Could you check a few things on this model? Use its own coordinates, in mm. A direction names the side the tool comes from. Round coordinates to 2 decimals unless told otherwise and drop trailing zeros. Loops run counter-clockwise (first coordinate to the right, second up) from the corner with the lowest first, then second, coordinate; pieces in that order, holes last.
from build123d import *

# Parameters (mm, degrees)
SKETCH1_W           = 100
SKETCH1_H           = 100
BOSS_EXTRUDE1_DEPTH = 10
SKETCH2_R           = 2.5
CUT_EXTRUDE1_DEPTH  = 30
SKETCH3_R           = 4
CUT_EXTRUDE2_DEPTH  = 10


with BuildPart() as part:
    # Sketch1 → Boss-Extrude1 (new body)
    with BuildSketch(Plane.XY):
        with Locations((50, 50)):
            Rectangle(SKETCH1_W, SKETCH1_H)
    extrude(amount=BOSS_EXTRUDE1_DEPTH)

    # Sketch2 → Cut-Extrude1 (cut)
    with BuildSketch(Plane.XZ):
        with Locations(Location((25, 5, 0), (0, 0, 270))):
            Circle(SKETCH2_R)
        with Locations(Location((50, 5, 0), (0, 0, 270))):
            Circle(SKETCH2_R)
        with Locations(Location((75, 5, 0), (0, 0, 270))):
            Circle(SKETCH2_R)
    extrude(amount=-CUT_EXTRUDE1_DEPTH, mode=Mode.SUBTRACT)

    # Sketch3 → Cut-Extrude2 (cut)
    with BuildSketch(Plane.XY.offset(10)):
        with Locations((90, 90)):
            Circle(SKETCH3_R)
        with Locations((90, 40)):
            Circle(SKETCH3_R)
    extrude(amount=-CUT_EXTRUDE2_DEPTH, mode=Mode.SUBTRACT)


solid = part.part
Item 1: We'd pull the mould along Y, two halves only. Please class faces 3 (the cylindrical face through (89.133, 86.095, 5.07)), 4 (the flat face through (49, 51, 0)), 5 (the flat face through (50, 30, 5)): released by +Y, released by -Y, zero draft, split by the parting line, or undercut.
Results list:
face 3: undercut
face 4: zero draft
face 5: released by -Y
Item 2: If we section it at D-D, the plane z = 5: Please give me the cut outline in (x, y).
Results list:
outline: (0, 0) - (22.5, 0) - (22.5, 30) - (27.5, 30) - (27.5, 0) - (47.5, 0) - (47.5, 30) - (52.5, 30) - (52.5, 0) - (72.5, 0) - (72.5, 30) - (77.5, 30) - (77.5, 0) - (100, 0) - (100, 100) - (0, 100) - close; hole circle Ø8 at (90, 40); hole circle Ø8 at (90, 90)
Item 3: Will this pin go through, and if not, where does the flat tip stop? pin 1 (1.5 mm diameter, centred on x = 25.5, z = 6, fed in from -Y).
Results list:
pin 1: stops at y = 30
Item 4: If we section it at A-A, the plane y = 90: Please give me the cut outline in (x, z).
Results list:
outline: (0, 0) - (86, 0) - (86, 10) - (0, 10) - close; (94, 0) - (100, 0) - (100, 10) - (94, 10) - close
Item 5: If we section it at C-C, the plane y = 20: Please give me the cut outline in (x, z).
Results list:
outline: (0, 0) - (100, 0) - (100, 10) - (0, 10) - close; hole circle Ø5 at (25, 5); hole circle Ø5 at (50, 5); hole circle Ø5 at (75, 5)
Item 6: If we section it at B-B, the plane x = 90: Please give me the cut outline in (y, z), then the cut area to 3 significant figures.
Results list:
outline: (0, 0) - (36, 0) - (36, 10) - (0, 10) - close; (44, 0) - (86, 0) - (86, 10) - (44, 10) - close; (94, 0) - (100, 0) - (100, 10) - (94, 10) - close
area: 840 mm2
Item 7: If I drill on line 1 along Y through (x, z) = (90, 5.5); line 2 along X through (y, z) = (23.75, 5); line 3 along X through (y, z) = (9, 6.75), over which ranges is the centre line in solid material (lowest first)?
Results list:
line 1: y = 0 to 36, 44 to 86, 94 to 100
line 2: x = 0 to 22.5, 27.5 to 47.5, 52.5 to 72.5, 77.5 to 100
line 3: x = 0 to 23.21, 26.79 to 48.21, 51.79 to 73.21, 76.79 to 100
Item 8: For faces 1 (the flat face through (49, 51, 10)), 2 (the cylindrical face through (27.11, 14.79, 3.66)), which set-ups out of +Z, -Z, +X, -X, +Y, -Y let a thin tool reach every point of the face, with its end or its side?
Results list:
face 1: +Z, +X, -X, +Y, -Y
face 2: -Y
